Geometry: final body of the model. Coordinates: model frame, mm. Face numbers are marked on the shaded views. A direction names the side the tool comes from. Coordinates: 2 decimals unless noted, no trailing zeros. Loops run counter-clockwise (first coordinate to the right, second up) from the corner with the lowest first, then second, coordinate; pieces in that order, holes last. Notation, with made-up numbers: (-20.75, -38) -> (19.25, -38) arc R27 cw to (19.25, -9) -> close; hole circle Ø5 at (33.25, 18). An arc over 180 degrees is marked (long way). One line per item, written item: value. Start each with the question number.
Item 1: Section query C-C on z = 13.5. Give the number of separate pieces and of enclosed holes in the cut face, then the cut area to 3 significant figures.
Item 2: Set-up query: the marked faces 1 and 2. Return all of +Z, -Z, +X, -X, +Y, -Y with unobstructed straight access to the full face (end or side cutting, diameter ignored); none if empty.
Item 3: Section query B-B on x = 10.5. Return loops of the section in (y, z).
Item 4: Mould query, pull axis Y, two halves, no side actions, for the marked faces 3, 4 and 5. Classes: +Y half, -Y half, draft (parallel to the pull), parting line (faces both ways), or undercut.
Item 5: Ray query, probe 1 along Y at (x, z) = (-19.5, 10); probe 2 along Y at (x, z) = (-42.8, 7.5); probe 3 along Y at (x, z) = (-34.35, 7.5). Return the intervals inside material, ascending. Write a range as from..to.
Item 6: Section query A-A on y = -44. Return loops of the section in (x, z), then the cut area to 3 significant figures.
Item 7: Contact query for flat-ended pins moving along their axis: pin 1 Ø8 at (y, z) = (-5, 8.5) entering from -X; pin 2 Ø6.5 at (y, z) = (-50.23, 7.5) entering from -X; pin 3 Ø7 at (y, z) = (-53, 10) entering from -X; pin 4 Ø2.5 at (x, y) = (-26.29, -27) entering from -Z. Output: stop coordinate, or through.
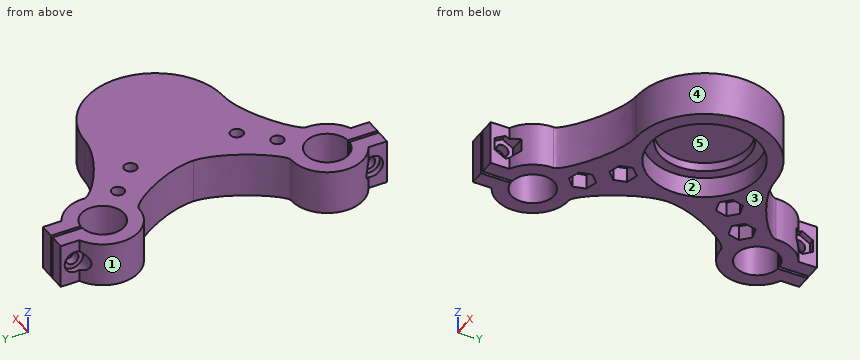
from build123d import *

# Parameters (mm, degrees)
SKETCH1_R               = 23.5
SKETCH1_R_2             = 18.5
BOSS_EXTRUDE1_DEPTH     = 7
SKETCH2_R               = 23.5
SKETCH2_R_2             = 15
BOSS_EXTRUDE2_DEPTH     = 3
SKETCH3_R               = 23.5
BOSS_EXTRUDE3_DEPTH     = 5
BOSS_EXTRUDE4_DEPTH     = 15
CUT_EXTRUDE1_DEPTH      = 88.358719822
CUT_EXTRUDE1_DEPTH_BACK = 88.358719822
SKETCH5_R               = 2.1
CUT_EXTRUDE2_DEPTH      = 88.35871984
CUT_EXTRUDE2_DEPTH_BACK = 2
SKETCH6_R               = 3.65
CUT_EXTRUDE3_DEPTH      = 80.375978306
CUT_EXTRUDE3_DEPTH_BACK = 2
BOSS_EXTRUDE6_START     = -15
BOSS_EXTRUDE6_DEPTH     = 15
SKETCH9_R               = 2.15
CUT_EXTRUDE4_DEPTH      = 15
CUT_EXTRUDE5_DEPTH      = 5
SKETCH11_W              = 94.20005325
SKETCH11_H              = 33.320618951
CUT_EXTRUDE6_DEPTH      = 25


# Read off the part's stored shape, not the designer's step: Boss-Extrude6
with BuildPart() as part:
    # Sketch1 → Boss-Extrude1 (new body)
    with BuildSketch(Plane.XY):
        Circle(SKETCH1_R)
        Circle(SKETCH1_R_2, mode=Mode.SUBTRACT)
    extrude(amount=BOSS_EXTRUDE1_DEPTH)

    # Sketch2 → Boss-Extrude2 (add)
    with BuildSketch(Plane.XY.offset(7)):
        Circle(SKETCH2_R)
        Circle(SKETCH2_R_2, mode=Mode.SUBTRACT)
    extrude(amount=BOSS_EXTRUDE2_DEPTH)

    # Sketch3 → Boss-Extrude3 (add)
    with BuildSketch(Plane.XY.offset(10)):
        Circle(SKETCH3_R)
    extrude(amount=BOSS_EXTRUDE3_DEPTH)



with BuildPart() as body_2:
    # Sketch4 → Boss-Extrude4 (new body)
    with BuildSketch(Plane.XY.offset(15)):
        with BuildLine():
            Line((-37.5, 45.221711778), (-37.5, 55.231747474))
            Line((-37.5, 55.231747474), (-42.5, 55.231747474))
            Line((-42.5, 55.231747474), (-42.5, 48.933577685))
            ThreePointArc((-42.5, 48.933577685), (-37, 25.761), (-31.5, 48.933577685))
            Line((-31.5, 48.933577685), (-31.5, 55.231747474))
            Line((-31.5, 55.231747474), (-36.5, 55.231747474))
            Line((-36.5, 55.231747474), (-36.5, 45.221711778))
            ThreePointArc((-36.5, 45.221711778), (-37, 30.761), (-37.5, 45.221711778))
        make_face()
    extrude(amount=-BOSS_EXTRUDE4_DEPTH)

    # Sketch5 → Cut-Extrude1 (cut, two sides: drawn at the far end of the back side and taken through both)
    with BuildSketch(Plane.ZY.offset(42.5).offset(-CUT_EXTRUDE1_DEPTH_BACK)):
        with Locations(Location((7.5, 50.231747474, 0), (0, 0, 321.816935122))):
            Circle(SKETCH5_R)
    extrude(amount=CUT_EXTRUDE1_DEPTH + CUT_EXTRUDE1_DEPTH_BACK, mode=Mode.SUBTRACT)

    # Sketch6 → Cut-Extrude2 (cut, two sides: drawn at the far end of the back side and taken through both)
    with BuildSketch(Plane.ZY.offset(42.5).offset(-CUT_EXTRUDE2_DEPTH_BACK)):
        with Locations(Location((7.5, 50.231747474, 0), (0, 0, 200.834080871))):
            Circle(SKETCH6_R)
    extrude(amount=CUT_EXTRUDE2_DEPTH + CUT_EXTRUDE2_DEPTH_BACK, mode=Mode.SUBTRACT)

    # Sketch7 → Cut-Extrude3 (cut, two sides: drawn at the far end of the back side and taken through both)
    with BuildSketch(Plane(origin=(-31.5, 0, 0), x_dir=(0, 0, -1), z_dir=(1, 0, 0)).offset(-CUT_EXTRUDE3_DEPTH_BACK)):
        Polygon((-5.392671517, 53.881747474), (-9.607328483, 53.881747474), (-11.714656965, 50.231747474), (-9.607328483, 46.581747474), (-5.392671517, 46.581747474), (-3.285343035, 50.231747474), align=None)
    extrude(amount=CUT_EXTRUDE3_DEPTH + CUT_EXTRUDE3_DEPTH_BACK, mode=Mode.SUBTRACT)


with BuildPart() as part_1:
    add(part.part)

    add(body_2.part)  # Boss-Extrude6 merges body 2
    # Boss-Extrude6 outline → Boss-Extrude6 (add)
    with BuildSketch(Plane.XY.offset(15).offset(BOSS_EXTRUDE6_START)):
        with BuildLine():
            ThreePointArc((-24.765350871, 37.673684678), (-28.461869415, 29.231109129), (-37, 25.761))
            add(Edge.make_bspline(
                [(-37, 25.761), (-34, 25.761), (-23.5, 10), (-23.5, 0)],
                knots=[0, 0, 0, 0, 1, 1, 1, 1], degree=3))
            ThreePointArc((-23.5, 0), (-16.393992054, 16.83707292), (0.626555279, 23.49164593))
            add(Edge.make_bspline(
                [(-24.765350871, 37.673684678), (-24.845336651, 34.674751155), (-9.369889797, 23.758265197), (0.626555279, 23.49164593)],
                knots=[0, 0, 0, 0, 1, 1, 1, 1], degree=3))
        make_face()
    extrude(amount=BOSS_EXTRUDE6_DEPTH)

    # Sketch9 → Cut-Extrude4 (cut)
    with BuildSketch(Plane.XY.offset(15)):
        with Locations((-17.526315789, 18)):
            Circle(SKETCH9_R)
        with Locations((-26.289473684, 27)):
            Circle(SKETCH9_R)
    extrude(amount=-CUT_EXTRUDE4_DEPTH, mode=Mode.SUBTRACT)

    # Sketch10 → Cut-Extrude5 (cut)
    with BuildSketch(Plane(origin=(0, 0, 0), x_dir=(-1, 0, 0), z_dir=(0, 0, -1))):
        Polygon((25.253012932, 22.914772657), (29.309153967, 24.059784987), (30.345614719, 28.14501233), (27.325934436, 31.085227343), (23.269793401, 29.940215013), (22.233332649, 25.85498767), align=None)
        Polygon((16.489855038, 13.914772657), (20.545996073, 15.059784987), (21.582456825, 19.14501233), (18.562776541, 22.085227343), (14.506635506, 20.940215013), (13.470174754, 16.85498767), align=None)
    extrude(amount=-CUT_EXTRUDE5_DEPTH, mode=Mode.SUBTRACT)

    # Sketch11 → Cut-Extrude6 (cut)
    with BuildSketch(Plane(origin=(0, 0, 0), x_dir=(1, 0, 0), z_dir=(0, 1, 0))):
        with Locations((-10.776769446, -9.973227019)):
            Rectangle(SKETCH11_W, SKETCH11_H)
    extrude(amount=-CUT_EXTRUDE6_DEPTH, mode=Mode.SUBTRACT)

    # Mirror4: part across plane


with BuildPart() as part_2:
    add(part_1.part)
    add(part_1.part.mirror(Plane.ZX))


solid = part_2.part
Reply:
1. separate pieces: 1
1. enclosed holes: 4
1. area: 3,150 mm²
2. face 1: +Z, -Z, -X
2. face 2: -Z
3. outline: (-21.02, 0) -> (-15.23, 0) -> (-15.23, 7) -> (-10.71, 7) -> (-10.71, 10) -> (10.71, 10) -> (10.71, 7) -> (15.23, 7) -> (15.23, 0) -> (21.02, 0) -> (21.02, 15) -> (-21.02, 15) -> close
4. face 3: draft
4. face 4: parting line
4. face 5: undercut
5. probe 1: y = -32.01..-18.85, -17.15..17.15, 18.85..32.01
5. probe 2: y = -46.58..-42.33, -33.67..-27.22, 27.22..33.67, 42.33..46.58
5. probe 3: y = -55.23..-52.33, -48.13..-44.74, -31.26..-23.94, 23.94..31.26, 44.74..48.13, 52.33..55.23
6. outline: (-47.67, 0) -> (-41.05, 0) -> (-41.05, 15) -> (-47.67, 15) -> close; (-32.95, 0) -> (-26.33, 0) -> (-26.33, 15) -> (-32.95, 15) -> close
6. area: 199 mm²
7. pin 1: stops at x = -25.47
7. pin 2: stops at x = -40.5
7. pin 3: stops at x = -42.5
7. pin 4: passes through
